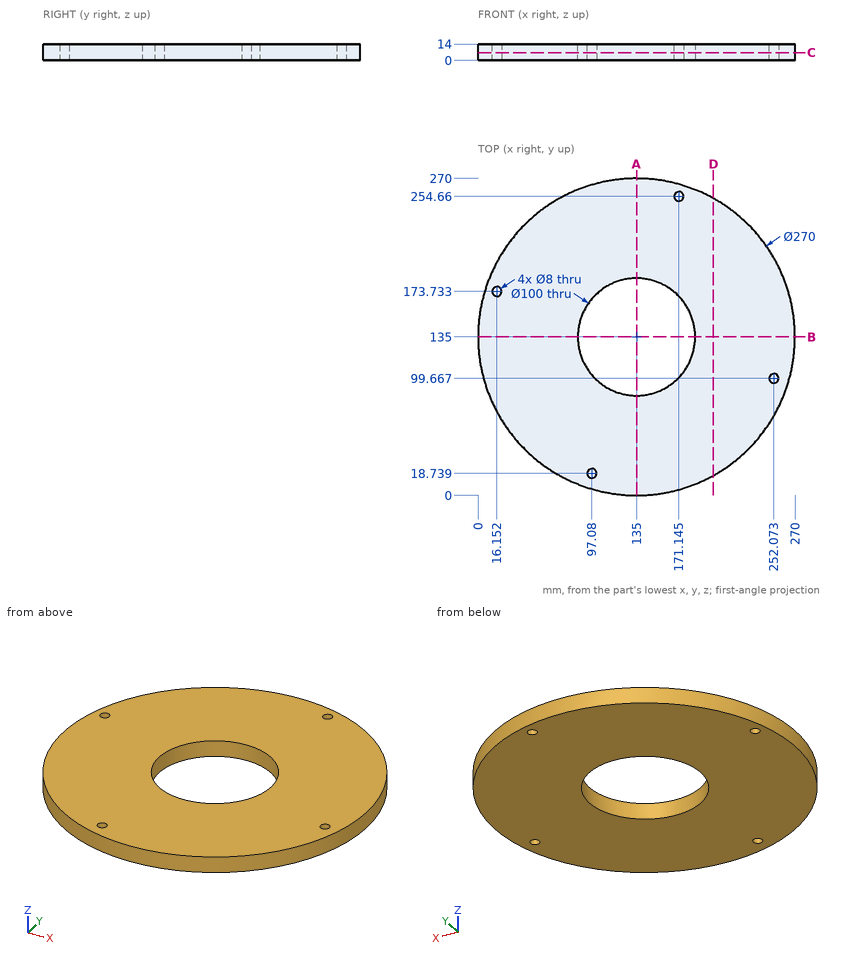
Geometry check sheet. Reference: drawing and pictorial views, mm from the part's lowest x, y, z. Give positions to 0.01 mm unless a question says otherwise; leave off trailing zeros. Order: outer loops, then holes, each group sorted by start corner. A loop starts at its lowest first (then second) coordinate and runs counter-clockwise, first axis right, second up. Notation, with made-up numbers: M 49.25,17.25 L 71.25,17.25 A24 ccw 71.25,46.25 Z; hole C -34,-20.5 d9. An arc over 180 degrees is marked long. Answer in a Markdown table with one row per item. Add a question column.
Item 1: Section check A-A, the plane x = 135. Enter the section's corners in (y, z).
Item 2: Section check C-C, the plane z = 6.75. Enter the section's corners in (x, y) (1 decimal), and give its area (3 significant figures).
Item 3: Section check D-D, the plane x = 200.5. Enter the section's corners in (y, z) (1 decimal).
Item 4: Scan lines: probe 1 along X at (y, z) = (173.5, 6) (1 decimal); probe 2 along Y at (x, z) = (135, 5.25); probe 3 along Y at (x, z) = (19, 7.5) (1 decimal). Record each from-to range of solid material in increasing order. Write a range as from..to.
Item 5: Gauge pin test, flat ends, axial feed: pin 1 (1.5 mm diameter, centred on x = 192.5, z = 5, fed in from +Y); pin 2 (1 mm diameter, centred on x = 53, z = 2.5, fed in from +Y); pin 3 (3 mm diameter, centred on y = 97.5, z = 7.5, fed in from -X). Record the tip position at first contact, or that the pin passes through.
Filled sheet:
| question | item | result |
|---|---|---|
| 1 | outline | M 0,0 L 85,0 L 85,14 L 0,14 Z; M 185,0 L 270,0 L 270,14 L 185,14 Z |
| 2 | outline | C 135,135 d270; hole C 16.2,173.7 d8; hole C 135,135 d100; hole C 97.1,18.7 d8; hole C 171.1,254.7 d8; hole C 252.1,99.7 d8 |
| 2 | area | 49,200 mm^2 |
| 3 | outline | M 17,0 L 253,0 L 253,14 L 17,14 Z |
| 4 | probe 1 | x = 5.6..12.2, 20.1..103.1, 166.9..264.4 |
| 4 | probe 2 | y = 0..85, 185..270 |
| 4 | probe 3 | y = 65.9..170.9, 176.5..204.1 |
| 5 | pin 1 | stops at y = 257.49 |
| 5 | pin 2 | stops at y = 242.62 |
| 5 | pin 3 | stops at x = 4.89 |
